```python
from build123d import *

# Parameters (mm, degrees)
ESBO_O1_W                      = 4
ESBO_O1_H                      = 4
RESSALTO_EXTRUS_O1_DEPTH       = 300
PADR_OCIRCULAR1_COUNT          = 4
PADR_O_LINEAR1_COUNT           = 2
PADR_O_LINEAR1_PITCH           = 30
PADR_O_LINEAR1_COPY_1_SKETCH_W = 4
PADR_O_LINEAR1_COPY_1_SKETCH_H = 4
PADR_O_LINEAR1_COPY_1_DEPTH    = 300
PADR_O_LINEAR1_COPY_2_SKETCH_W = 4
PADR_O_LINEAR1_COPY_2_SKETCH_H = 4
PADR_O_LINEAR1_COPY_2_DEPTH    = 300
PADR_O_LINEAR1_COPY_3_SKETCH_W = 4
PADR_O_LINEAR1_COPY_3_SKETCH_H = 4
PADR_O_LINEAR1_COPY_3_DEPTH    = 300
ESBO_O4_W                      = 10
ESBO_O4_H                      = 28
CORTE_EXTRUS_O1_DEPTH          = 304.72685097
FILETE1_R                      = 1
SKETCH1_R                      = 2.5
CUT_EXTRUDE1_DEPTH             = 3
SKETCH2_R                      = 4
CUT_EXTRUDE2_DEPTH             = 305.836021494


with BuildPart() as part:
    # Esboço1 → Ressalto-extrusão1 (new body)
    with BuildSketch(Plane.XY):
        with BuildLine():
            ThreePointArc((-1.664601464, 3.078815026), (-0.858529967, 3.393070335), (0, 3.5))
            Line((0, 3.5), (0, 6))
            Line((0, 6), (-3.878679656, 6))
            Line((-3.878679656, 6), (-8.5, 10.621320344))
            Line((-8.5, 10.621320344), (-8.5, 13))
            Line((-8.5, 13), (-4.1, 13))
            Line((-4.1, 13), (-4.1, 14.5))
            Line((-4.1, 14.5), (-5.1, 14.5))
            Line((-5.1, 14.5), (-5.1, 15))
            Line((-5.1, 15), (-15, 15))
            Line((-15, 15), (-15, 5.1))
            Line((-15, 5.1), (-14.5, 5.1))
            Line((-14.5, 5.1), (-14.5, 4.1))
            Line((-14.5, 4.1), (-13, 4.1))
            Line((-13, 4.1), (-13, 8.5))
            Line((-13, 8.5), (-10.621320344, 8.5))
            Line((-10.621320344, 8.5), (-6, 3.878679656))
            Line((-6, 3.878679656), (-6, 0))
            Line((-6, 0), (-3.5, 0))
            ThreePointArc((-3.5, 0), (-3.393070335, 0.858529967), (-3.078815026, 1.664601464))
            Line((-3.078815026, 1.664601464), (-4.596194078, 3.181980515))
            Line((-4.596194078, 3.181980515), (-3.181980515, 4.596194078))
            Line((-3.181980515, 4.596194078), (-1.664601464, 3.078815026))
        make_face()
        with Locations((-12, 12)):
            Rectangle(ESBO_O1_W, ESBO_O1_H, mode=Mode.SUBTRACT)
    ressalto_extrus_o1 = extrude(amount=RESSALTO_EXTRUS_O1_DEPTH)

    # PadrãoCircular1: Ressalto-extrusão1 ×4 about axis
    padr_ocircular1_axis = Axis((0, 0, 0), (0, 0, 1))
    for i in range(1, PADR_OCIRCULAR1_COUNT):
        add(ressalto_extrus_o1.rotate(padr_ocircular1_axis, i * 360 / PADR_OCIRCULAR1_COUNT))

    # Padrão linear1: Ressalto-extrusão1 ×2
    with Locations(*[(i * PADR_O_LINEAR1_PITCH, 0, 0) for i in range(1, PADR_O_LINEAR1_COUNT)]):
        add(ressalto_extrus_o1)

    # Padrão linear1 copy 1 sketch → Padrão linear1 copy 1 (add)
    with BuildSketch(Plane(origin=(30, 0, 0), x_dir=(0, 1, 0), z_dir=(0, 0, 1))):
        with BuildLine():
            ThreePointArc((-1.664601464, 3.078815026), (-0.858529967, 3.393070335), (0, 3.5))
            Line((0, 3.5), (0, 6))
            Line((0, 6), (-3.878679656, 6))
            Line((-3.878679656, 6), (-8.5, 10.621320344))
            Line((-8.5, 10.621320344), (-8.5, 13))
            Line((-8.5, 13), (-4.1, 13))
            Line((-4.1, 13), (-4.1, 14.5))
            Line((-4.1, 14.5), (-5.1, 14.5))
            Line((-5.1, 14.5), (-5.1, 15))
            Line((-5.1, 15), (-15, 15))
            Line((-15, 15), (-15, 5.1))
            Line((-15, 5.1), (-14.5, 5.1))
            Line((-14.5, 5.1), (-14.5, 4.1))
            Line((-14.5, 4.1), (-13, 4.1))
            Line((-13, 4.1), (-13, 8.5))
            Line((-13, 8.5), (-10.621320344, 8.5))
            Line((-10.621320344, 8.5), (-6, 3.878679656))
            Line((-6, 3.878679656), (-6, 0))
            Line((-6, 0), (-3.5, 0))
            ThreePointArc((-3.5, 0), (-3.393070335, 0.858529967), (-3.078815026, 1.664601464))
            Line((-3.078815026, 1.664601464), (-4.596194078, 3.181980515))
            Line((-4.596194078, 3.181980515), (-3.181980515, 4.596194078))
            Line((-3.181980515, 4.596194078), (-1.664601464, 3.078815026))
        make_face()
        with Locations((-12, 12)):
            Rectangle(PADR_O_LINEAR1_COPY_1_SKETCH_W, PADR_O_LINEAR1_COPY_1_SKETCH_H, mode=Mode.SUBTRACT)
    extrude(amount=PADR_O_LINEAR1_COPY_1_DEPTH)

    # Padrão linear1 copy 2 sketch → Padrão linear1 copy 2 (add)
    with BuildSketch(Plane(origin=(30, 0, 0), x_dir=(-1, 0, 0), z_dir=(0, 0, 1))):
        with BuildLine():
            ThreePointArc((-1.664601464, 3.078815026), (-0.858529967, 3.393070335), (0, 3.5))
            Line((0, 3.5), (0, 6))
            Line((0, 6), (-3.878679656, 6))
            Line((-3.878679656, 6), (-8.5, 10.621320344))
            Line((-8.5, 10.621320344), (-8.5, 13))
            Line((-8.5, 13), (-4.1, 13))
            Line((-4.1, 13), (-4.1, 14.5))
            Line((-4.1, 14.5), (-5.1, 14.5))
            Line((-5.1, 14.5), (-5.1, 15))
            Line((-5.1, 15), (-15, 15))
            Line((-15, 15), (-15, 5.1))
            Line((-15, 5.1), (-14.5, 5.1))
            Line((-14.5, 5.1), (-14.5, 4.1))
            Line((-14.5, 4.1), (-13, 4.1))
            Line((-13, 4.1), (-13, 8.5))
            Line((-13, 8.5), (-10.621320344, 8.5))
            Line((-10.621320344, 8.5), (-6, 3.878679656))
            Line((-6, 3.878679656), (-6, 0))
            Line((-6, 0), (-3.5, 0))
            ThreePointArc((-3.5, 0), (-3.393070335, 0.858529967), (-3.078815026, 1.664601464))
            Line((-3.078815026, 1.664601464), (-4.596194078, 3.181980515))
            Line((-4.596194078, 3.181980515), (-3.181980515, 4.596194078))
            Line((-3.181980515, 4.596194078), (-1.664601464, 3.078815026))
        make_face()
        with Locations((-12, 12)):
            Rectangle(PADR_O_LINEAR1_COPY_2_SKETCH_W, PADR_O_LINEAR1_COPY_2_SKETCH_H, mode=Mode.SUBTRACT)
    extrude(amount=PADR_O_LINEAR1_COPY_2_DEPTH)

    # Padrão linear1 copy 3 sketch → Padrão linear1 copy 3 (add)
    with BuildSketch(Plane(origin=(30, 0, 0), x_dir=(0, -1, 0), z_dir=(0, 0, 1))):
        with BuildLine():
            ThreePointArc((-1.664601464, 3.078815026), (-0.858529967, 3.393070335), (0, 3.5))
            Line((0, 3.5), (0, 6))
            Line((0, 6), (-3.878679656, 6))
            Line((-3.878679656, 6), (-8.5, 10.621320344))
            Line((-8.5, 10.621320344), (-8.5, 13))
            Line((-8.5, 13), (-4.1, 13))
            Line((-4.1, 13), (-4.1, 14.5))
            Line((-4.1, 14.5), (-5.1, 14.5))
            Line((-5.1, 14.5), (-5.1, 15))
            Line((-5.1, 15), (-15, 15))
            Line((-15, 15), (-15, 5.1))
            Line((-15, 5.1), (-14.5, 5.1))
            Line((-14.5, 5.1), (-14.5, 4.1))
            Line((-14.5, 4.1), (-13, 4.1))
            Line((-13, 4.1), (-13, 8.5))
            Line((-13, 8.5), (-10.621320344, 8.5))
            Line((-10.621320344, 8.5), (-6, 3.878679656))
            Line((-6, 3.878679656), (-6, 0))
            Line((-6, 0), (-3.5, 0))
            ThreePointArc((-3.5, 0), (-3.393070335, 0.858529967), (-3.078815026, 1.664601464))
            Line((-3.078815026, 1.664601464), (-4.596194078, 3.181980515))
            Line((-4.596194078, 3.181980515), (-3.181980515, 4.596194078))
            Line((-3.181980515, 4.596194078), (-1.664601464, 3.078815026))
        make_face()
        with Locations((-12, 12)):
            Rectangle(PADR_O_LINEAR1_COPY_3_SKETCH_W, PADR_O_LINEAR1_COPY_3_SKETCH_H, mode=Mode.SUBTRACT)
    extrude(amount=PADR_O_LINEAR1_COPY_3_DEPTH)

    # Esboço4 → Corte-extrusão1 (cut, through all)
    with BuildSketch(Plane(origin=(0, 0, 0), x_dir=(-1, 0, 0), z_dir=(0, 0, -1))):
        with Locations((-15, 0)):
            Rectangle(ESBO_O4_W, ESBO_O4_H)
    extrude(amount=-CORTE_EXTRUS_O1_DEPTH, mode=Mode.SUBTRACT)

    # Filete1
    filete1_edges = [part.edges().sort_by_distance(p)[0] for p in [
        (45, -15, 150),
        (45, 15, 150),
        (-15, 15, 150),
        (-15, -15, 150),
    ]]
    fillet(filete1_edges, radius=FILETE1_R)

    # Sketch1 → Cut-Extrude1 (cut)
    with BuildSketch(Plane(origin=(0, 15, 0), x_dir=(1, 0, 0), z_dir=(0, 1, 0))):
        with BuildLine():
            ThreePointArc((19, -150), (17.54586978, -146.914785735), (14.24072647, -146.072723118))
            Line((14.24072647, -146.072723118), (15.75927353, -153.927276882))
            ThreePointArc((15.75927353, -153.927276882), (18.085214265, -152.54586978), (19, -150))
        make_face()
        with BuildLine():
            Line((15.75927353, -153.927276882), (14.24072647, -146.072723118))
            ThreePointArc((14.24072647, -146.072723118), (11.072723118, -150.75927353), (15.75927353, -153.927276882))
        make_face()
        with Locations((33.25, -150)):
            Circle(SKETCH1_R)
        with Locations((-3.25, -150)):
            Circle(SKETCH1_R)
    extrude(amount=-CUT_EXTRUDE1_DEPTH, mode=Mode.SUBTRACT)

    # Sketch2 → Cut-Extrude2 (cut, through all)
    with BuildSketch(Plane(origin=(0, 15, 0), x_dir=(1, 0, 0), z_dir=(0, 1, 0))):
        with Locations(Location((15, -150, 0), (0, 0, 180))):
            Circle(SKETCH2_R)
    extrude(amount=-CUT_EXTRUDE2_DEPTH, mode=Mode.SUBTRACT)


solid = part.part
```
Geometry check sheet. Reference: the model listing, model coordinates, mm. A direction names the side the tool comes from. Round coordinates to 2 decimals unless told otherwise and drop trailing zeros. Write item = value, one per line. Start each with the question number.
1. Section check A-A on z = 228.5. Give the number of separate pieces and of enclosed holes in the cut face, then the cut area to 3 significant figures.
2. Thickness scan on line 1 (Y direction, x = 41, z = 277.5); line 2 (X direction, y = -11, z = 246); line 3 (X direction, y = 6.25, z = 264). Record the ranges inside material, lowest first.
3. Depth check by flat-ended pin: pin 1 (0.5 mm diameter, centred on x = -4.5, z = 256.5, fed in from +Y); pin 2 (3 mm diameter, centred on y = 2, z = 62.5, fed in from -X); pin 3 (0.6 mm diameter, centred on y = 14.5, z = 233, fed in from -X); pin 4 (1.5 mm diameter, centred on x = -5.5, y = -11.5, fed in from -Z). Enter the tip coordinate at first touch or a pass-through.
4. Mould release check, pull along X, two halves, no side actions. Record for faces 6 (the face through (39, -15, 148)), 7 (the face through (-15, 10, 148)), 8 (the face through (45, -10, 148)), 9 (the face through (-8.34, 6.22, 147.9)): released by +X, released by -X, zero draft, split by the parting line, or undercut.
5. Set-up check for faces 1 (the face through (-15, -9, 148)), 2 (the face through (30, -6, 148)), 3 (the face through (-6, 0, 148)), 4 (the face through (20, 15, 148)), 5 (the face through (36.22, 8.34, 147.9)): record each of +Z, -Z, +X, -X, +Y, -Y from which the full face is reachable in a straight line by a thin tool's end or side.
Working result:
q1.separate_pieces = 1
q1.enclosed_holes = 7
q1.area = 561 mm^2
q2.line_1 = -15 to -14, -10 to -8.5, 8.5 to 10, 14 to 15
q2.line_2 = -15 to -14, -10 to -8.5, 8.5 to 10, 20 to 21.5, 38.5 to 40, 44 to 45
q2.line_3 = -15 to -13, -8.37 to -4.13, 4.13 to 8.37, 21.63 to 25.87, 34.13 to 38.37, 43 to 45
q3.pin_1 = 14.5
q3.pin_2 = -6
q3.pin_3 = -14.98
q3.pin_4 = through
q4.face_6 = zero draft
q4.face_7 = released by -X
q4.face_8 = released by +X
q4.face_9 = undercut
q5.face_1 = +Z, -Z, -X, +Y, -Y
q5.face_2 = +Z, -Z, -Y
q5.face_3 = +Z, -Z, -X
q5.face_4 = +Z, -Z, +X, -X, +Y
q5.face_5 = +Z, -Z
